```python
from build123d import *

# Parameters (mm, degrees)
SKETCH_1_W                  = 40
SKETCH_1_H                  = 40
SKETCH_1_W_2                = 32
SKETCH_1_H_2                = 32
EXTRUDE_1_DEPTH             = 396
HOLE_WIZARD_M61_D           = 5
HOLE_WIZARD_M61_DEPTH       = 17
HOLE_WIZARD_M61_CSINK_D     = 6.05
HOLE_WIZARD_M61_CSINK_ANGLE = 120
HOLE_WIZARD_M61_TIP         = 1.502151548
HOLE_WIZARD_M41_D           = 3.3
HOLE_WIZARD_M41_DEPTH       = 11.5
HOLE_WIZARD_M41_CSINK_D     = 4.05
HOLE_WIZARD_M41_CSINK_ANGLE = 120
HOLE_WIZARD_M41_TIP         = 0.991420021


with BuildPart() as part:
    # Эскиз1 → Вытянуть-Тонкостенный1 (new body)
    with BuildSketch(Plane.XY):
        with Locations((20, 20)):
            Rectangle(SKETCH_1_W, SKETCH_1_H)
        with Locations((20, 20)):
            Rectangle(SKETCH_1_W_2, SKETCH_1_H_2, mode=Mode.SUBTRACT)
    extrude(amount=EXTRUDE_1_DEPTH)

    # Отверстие обработанное метчиком M61
    with Locations(Plane.ZY):
        with Locations((30, 20), (80, 20), (130, 20), (180, 20), (230, 20), (280, 20), (330, 20)):
            CounterSinkHole(HOLE_WIZARD_M61_D / 2, HOLE_WIZARD_M61_CSINK_D / 2, depth=HOLE_WIZARD_M61_DEPTH, counter_sink_angle=HOLE_WIZARD_M61_CSINK_ANGLE)
            with Locations((0, 0, -(HOLE_WIZARD_M61_DEPTH + HOLE_WIZARD_M61_TIP / 2))):  # 118° drill point
                Cone(0, HOLE_WIZARD_M61_D / 2, HOLE_WIZARD_M61_TIP, mode=Mode.SUBTRACT)

    # Отверстие обработанное метчиком M41
    with Locations(Plane.ZY):
        with Locations((386, 10), (366, 10), (386, 30), (366, 30)):
            CounterSinkHole(HOLE_WIZARD_M41_D / 2, HOLE_WIZARD_M41_CSINK_D / 2, depth=HOLE_WIZARD_M41_DEPTH, counter_sink_angle=HOLE_WIZARD_M41_CSINK_ANGLE)
            with Locations((0, 0, -(HOLE_WIZARD_M41_DEPTH + HOLE_WIZARD_M41_TIP / 2))):  # 118° drill point
                Cone(0, HOLE_WIZARD_M41_D / 2, HOLE_WIZARD_M41_TIP, mode=Mode.SUBTRACT)


solid = part.part
```
CAD build for the part. Positions are in the model's coordinates, mm. A direction names the side the tool comes from. Give positions to 0.01 mm unless a question says otherwise; leave off trailing zeros. Order: outer loops, then holes, each group sorted by start corner. A loop starts at its lowest first (then second) coordinate and runs counter-clockwise, first axis right, second up.
(1) Saw through at B-B, the plane x = 16.5. Give the cut face in (y, z).
(2) Drill centre lines: L1, parallel to Z at x = 2.85, y = 30; L2, parallel to Y at x = 34, z = 374. Where is each one in solid material? Low to high.
(3) Saw through at A-A, the plane z = 244. Give the cut face in (x, y).
(4) Tool access for faces 1 (the flat face through (2, 20, 0)), 2 (the flat face through (20, 4, 195)): list every direction of +Z, -Z, +X, -X, +Y, -Y with a clear straight run to the whole face (end or side of a thin tool).
(5) Flat gauge pins, fed straight in: pin 1 (9.5 mm diameter, centred on x = 25, z = 198.5, fed in from -Y); pin 2 (4.5 mm diameter, centred on y = 20, z = 330, fed in from -X); pin 3 (6 mm diameter, centred on y = 20, z = 230, fed in from -X). Where does each tip first touch, or does it go through?
Results found:
1. outline: (0, 0) - (4, 0) - (4, 396) - (0, 396) - close; (36, 0) - (40, 0) - (40, 396) - (36, 396) - close
2. L1: z = 0 to 364.35, 367.65 to 384.35, 387.65 to 396
2. L2: y = 0 to 4, 36 to 40
3. outline: (0, 0) - (40, 0) - (40, 40) - (0, 40) - close; hole (4, 4) - (36, 4) - (36, 36) - (4, 36) - close
4. face 1: -Z, +X, -X, +Y, -Y
4. face 2: +Z, -Z
5. pin 1: stops at y = 0
5. pin 2: stops at x = 36
5. pin 3: stops at x = 0.01
